The model under review builds one solid part; all positions refer to its coordinate system, in mm. A direction names the side the tool comes from. Round coordinates to 2 decimals unless told otherwise and drop trailing zeros. Loops run counter-clockwise (first coordinate to the right, second up) from the corner with the lowest first, then second, coordinate; pieces in that order, holes last. Notation, with made-up numbers: M 8.25,33 L 54.25,33 A17 cw 54.25,44 Z; hole C -8,18.5 d4. An arc over 180 degrees is marked long. One line per question, with ' | ' between items.
from build123d import *

# Parameters (mm, degrees)
BOSS_EXTRUDE1_DEPTH = 15


with BuildPart() as part:
    # Sketch1 → Boss-Extrude1 (new body)
    with BuildSketch(Plane(origin=(0, 0, 0), x_dir=(1, 0, 0), z_dir=(0, 1, 0))):
        with BuildLine():
            Line((15.892322519, -36.707411853), (9.932701575, -22.942132408))
            Line((9.932701575, -22.942132408), (-0.134306126, -27.300601859))
            Line((-0.134306126, -27.300601859), (5.215978235, -39.658461532))
            ThreePointArc((5.215978235, -39.658461532), (10.656794252, -38.554282982), (15.892322519, -36.707411853))
        make_face()
        with BuildLine():
            Line((40, 0), (25, 0))
            ThreePointArc((25, 0), (20.896381737, -13.723746949), (9.932701575, -22.942132408))
            Line((9.932701575, -22.942132408), (15.892322519, -36.707411853))
            ThreePointArc((15.892322519, -36.707411853), (33.434210779, -21.957995118), (40, 0))
        make_face()
        with BuildLine():
            Line((25, 7.62), (25, 0))
            Line((25, 0), (40, 0))
            ThreePointArc((40, 0), (39.816450827, 3.827563654), (39.267487824, 7.62))
            Line((39.267487824, 7.62), (25, 7.62))
        make_face()
        with BuildLine():
            Line((5.825314819, -41.065881304), (15.892322519, -36.707411853))
            ThreePointArc((15.892322519, -36.707411853), (10.656794252, -38.554282982), (5.215978235, -39.658461532))
            Line((5.215978235, -39.658461532), (5.825314819, -41.065881304))
        make_face()
        with BuildLine():
            ThreePointArc((39.267487824, 7.62), (39.816450827, 3.827563654), (40, 0))
            Line((40, 0), (40, 7.62))
            Line((40, 7.62), (39.267487824, 7.62))
        make_face()
    extrude(amount=BOSS_EXTRUDE1_DEPTH)


solid = part.part
1) Add section B-B on z = 26. State the section outline as (x, y) points, then the cut area to 3 significant figures.
Output values:
outline: M 2.87,0 L 30.4,0 L 30.4,15 L 2.87,15 Z | area: 413 mm²
2) Add section C-C on x = 13.5. State the section outline as (y, z) points, then the cut area to 3 significant figures.
Output values:
outline: M 0,21.04 L 15,21.04 L 15,37.74 L 0,37.74 Z | area: 251 mm²
3) Add section A-A on y = 14.25. State the section outline as (x, z) points, then the cut area to 3 significant figures.
Output values:
outline: M -0.13,27.3 L 9.93,22.94 A25 cw 25,0 L 25,-7.62 L 40,-7.62 L 40,0 A40 ccw 15.89,36.71 L 5.83,41.07 Z | area: 845 mm²
4) Machinability: for faces 1 (the flat face through (25, 7, -4)), 2 (the flat face through (24, 0, 16)), which of the approach directions +Z, -Z, +X, -X, +Y, -Y give a long, thin tool a straight path to every point of the face, cutting with its end or side? Answer none if there is none.
Output values:
face 1: -Z, -X, +Y, -Y | face 2: +Z, -Z, +X, -X, -Y
5) Insertion check: P1, Ø5, axis at y = 1.5, z = 24, coming from the +X side; P2, Ø5, axis at y = 3, z = 29.5, coming from the +X side; P3, Ø1, axis at x = 28, y = 4, coming from the +Z side. Each pin has a flat end and moves straight along its axis. Give the tip position at first contact, or say it passes through.
Output values:
P1: stops at x = 33.73 | P2: stops at x = 29.51 | P3: stops at z = 29.05
6) For line 1 (Z direction, x = 29.5, y = 8.5); line 2 (Z direction, x = 20, y = 1.25); line 3 (X direction, y = 3.25, z = 16), list the stretches that pass through material, from the lowest coordinate up.
Output values:
line 1: z = -7.62 to 27.01 | line 2: z = 15 to 34.64 | line 3: x = 19.21 to 36.66
